Geometry check sheet. Reference: the model listing, model coordinates, mm. A direction names the side the tool comes from. Coordinates: 2 decimals unless noted, no trailing zeros. Order: outer loops, then holes, each group sorted by start corner. A loop starts at its lowest first (then second) coordinate and runs counter-clockwise, first axis right, second up. Notation, with made-up numbers: M 59.25,-28 L 86.25,-28 A19 cw 86.25,-1 Z; hole C 42.5,60 d1. An arc over 180 degrees is marked long. One line per item, written item: value. Start each with the question number.
1) Sectioned sample at B-B, the plane y = 107. Enter the section's corners in (x, z), then the cut area to 3 significant figures.
2) Go/stop test with flat-tipped pins: P1, Ø8.5, axis at x = 22.37, y = 47.5, coming from the +Z side; P2, Ø4, axis at x = 21.5, y = 47, coming from the +Z side; P3, Ø3, axis at y = 26, z = -41.5, coming from the -X side; P4, Ø2, axis at x = -45.13, z = -49.4, coming from the +Y side. Record where each tip stops, or that it passes through.
3) Thickness scan on L1, parallel to X at y = 6.5, z = -19.5; L2, parallel to X at y = 23, z = -22; L3, parallel to X at y = 47, z = -58. Record the ranges inside material, lowest first. Write a range as from..to.
4) Sectioned sample at A-A, the plane z = -35. State how many separate pieces and enclosed holes the cut face has, then the cut area to 3 significant figures.
5) Access from +Z, -Z, +X, -X, +Y, -Y to the whole of each face (thin tool, end or side, straight path). Record for faces 5 (the flat face through (-58.627, 44, -44)), 6 (the flat face through (21, 124, -55.901)), 7 (the flat face through (-66.627, 46, -43)), 8 (the flat face through (-63, 97, -49.401)).
6) Sectioned sample at D-D, the plane y = 18.5. Enter the section's corners in (x, z), then the cut area to 3 significant figures.
7) Draft check along Y on faces 1 (the flat face through (-16.7, -1.5, 7.1)), 2 (the flat face through (-64, 124, -55.901)), 3 (the flat face through (22, 97, -49.401)), 4 (the flat face through (-43, -10, -40)). Enter one of: pulls with the +Y half, pulls with the -Y half, needs draft (parallel to the pull), parting line crosses it, or undercut.
8) Sectioned sample at C-C, the plane x = -9. Enter the section's corners in (y, z), then the cut area to 3 significant figures.
```python
from build123d import *

# Parameters (mm, degrees)
SKETCH1_W           = 100
SKETCH1_H           = 70
SKETCH1_R           = 1.375
SKETCH1_R_2         = 27.5
BOSS_EXTRUDE1_DEPTH = 10
SKETCH3_W           = 8
SKETCH3_H           = 70
BOSS_EXTRUDE2_DEPTH = 55
CHAMFER1_SIZE       = 60
CHAMFER2_SIZE       = 3.5
SKETCH5_W           = 8
SKETCH5_H           = 10
BOSS_EXTRUDE3_DEPTH = 85
CUT_EXTRUDE1_START  = -3.5
SKETCH4_R           = 2.6
CUT_EXTRUDE1_DEPTH  = 169.016070813
SKETCH4_3_R         = 1.375
CUT_EXTRUDE2_DEPTH  = 172.516070813
CHAMFER3_SIZE       = 1


with BuildPart() as part:
    # Sketch1 → Boss-Extrude1 (new body)
    with BuildSketch(Plane(origin=(0, 0, 0), x_dir=(1, 0, 0), z_dir=(0, 1, 0))):
        with Locations((-20.126760563, 24.401408451)):
            Rectangle(SKETCH1_W, SKETCH1_H)
        with Locations(Location((-45.126760563, 49.401408451, 0), (0, 0, 270))):
            Circle(SKETCH1_R, mode=Mode.SUBTRACT)
        with Locations(Location((4.873239437, 49.401408451, 0), (0, 0, 270))):
            Circle(SKETCH1_R, mode=Mode.SUBTRACT)
        with Locations(Location((4.873239437, -0.598591549, 0), (0, 0, 270))):
            Circle(SKETCH1_R, mode=Mode.SUBTRACT)
        with Locations(Location((-45.126760563, -0.598591549, 0), (0, 0, 270))):
            Circle(SKETCH1_R, mode=Mode.SUBTRACT)
        with Locations(Location((-20.126760563, 24.401408451, 0), (0, 0, 270))):
            Circle(SKETCH1_R_2, mode=Mode.SUBTRACT)
    extrude(amount=-BOSS_EXTRUDE1_DEPTH)

    # Sketch3 → Boss-Extrude2 (add)
    with BuildSketch(Plane(origin=(0, 0, 0), x_dir=(1, 0, 0), z_dir=(0, 1, 0))):
        with Locations((-62.626760563, 24.401408451)):
            Rectangle(SKETCH3_W, SKETCH3_H)
        with Locations((22.373239437, 24.401408451)):
            Rectangle(SKETCH3_W, SKETCH3_H)
    extrude(amount=BOSS_EXTRUDE2_DEPTH)

    # Chamfer1
    chamfer1_edges = [part.edges().sort_by_distance(p)[0] for p in [
        (-62.626760563, 55, 10.598591549),
    ]]
    chamfer(chamfer1_edges, length=CHAMFER1_SIZE)

    # Chamfer2
    chamfer2_edges = [part.edges().sort_by_distance(p)[0] for p in [
        (26.373239437, 0, -26.901408451),
        (-66.626760563, 0, -26.901408451),
    ]]
    chamfer(chamfer2_edges, length=CHAMFER2_SIZE - 0.0001)  # a hair under: the kernel refuses the full size

    # Sketch5 → Boss-Extrude3 (add)
    with BuildSketch(Plane(origin=(0, 55, 0), x_dir=(1, 0, 0), z_dir=(0, 1, 0))):
        with Locations((-62.626760563, 54.401408451)):
            Rectangle(SKETCH5_W, SKETCH5_H)
        with Locations((22.373239437, 54.401408451)):
            Rectangle(SKETCH5_W, SKETCH5_H)
    extrude(amount=BOSS_EXTRUDE3_DEPTH)

    # Sketch4 → Cut-Extrude1 (cut, through all)
    with BuildSketch(Plane(origin=(0, 0, -59.401408451), x_dir=(-1, 0, 0), z_dir=(0, 0, -1)).offset(CUT_EXTRUDE1_START)):
        with Locations((-22.373239437, 47.5)):
            Circle(SKETCH4_R)
        with Locations((62.626760563, 47.5)):
            Circle(SKETCH4_R)
        with Locations((62.626760563, 7.5)):
            Circle(SKETCH4_R)
        with Locations((-22.373239437, 7.5)):
            Circle(SKETCH4_R)
        with Locations((-22.373239437, 125)):
            Circle(SKETCH4_R)
        with Locations((62.626760563, 125)):
            Circle(SKETCH4_R)
    extrude(amount=-CUT_EXTRUDE1_DEPTH, mode=Mode.SUBTRACT)

    # Sketch4<3> → Cut-Extrude2 (cut, through all)
    with BuildSketch(Plane(origin=(0, 0, -59.401408451), x_dir=(-1, 0, 0), z_dir=(0, 0, -1))):
        with Locations((-22.373239437, 47.5)):
            Circle(SKETCH4_3_R)
        with Locations((-22.373239437, 7.5)):
            Circle(SKETCH4_3_R)
        with Locations((62.626760563, 47.5)):
            Circle(SKETCH4_3_R)
        with Locations((62.626760563, 7.5)):
            Circle(SKETCH4_3_R)
        with Locations((-22.373239437, 125)):
            Circle(SKETCH4_3_R)
        with Locations((62.626760563, 125)):
            Circle(SKETCH4_3_R)
    extrude(amount=-CUT_EXTRUDE2_DEPTH, mode=Mode.SUBTRACT)

    # Chamfer3
    chamfer3_edges = [part.edges().sort_by_distance(p)[0] for p in [
        (-66.626760563, 29.24995, -23.651358451),
        (-66.626760563, 97.5, -49.401408451),
        (-58.626760563, 97.5, -49.401408451),
        (26.373239437, 97.5, -49.401408451),
        (18.373239437, 97.5, -49.401408451),
        (26.373239437, 29.24995, -23.651358451),
        (18.373239437, 27.5, -21.901408451),
        (-58.626760563, 27.5, -21.901408451),
    ]]
    chamfer(chamfer3_edges, length=CHAMFER3_SIZE)


solid = part.part
```
Final values:
1. outline: M -66.63,-59.4 L -58.63,-59.4 L -58.63,-50.4 L -59.63,-49.4 L -65.63,-49.4 L -66.63,-50.4 Z; M 18.37,-59.4 L 26.37,-59.4 L 26.37,-50.4 L 25.37,-49.4 L 19.37,-49.4 L 18.37,-50.4 Z
1. area: 158 mm^2
2. P1: stops at z = -37.65
2. P2: stops at z = -39.4
2. P3: stops at x = -66.63
2. P4: passes through
3. L1: x = -66.63..-65.03, -60.23..-58.63, 18.37..19.97, 24.77..26.37
3. L2: x = -66.63..-58.63, 18.37..26.37
3. L3: x = -66.63..-63.91, -61.35..-58.63, 18.37..21.09, 23.65..26.37
4. separate pieces: 2
4. enclosed holes: 2
4. area: 1,110 mm^2
5. face 5: +Z, -Z, +Y
5. face 6: +Z
5. face 7: +Z, -Z, -X, +Y
5. face 8: +Z, +X, -X, +Y
6. outline: M -66.63,-59.4 L -58.63,-59.4 L -58.63,-14.32 L -59.63,-12.9 L -65.63,-12.9 L -66.63,-14.32 Z; M 18.37,-59.4 L 26.37,-59.4 L 26.37,-14.32 L 25.37,-12.9 L 19.37,-12.9 L 18.37,-14.32 Z
6. area: 741 mm^2
7. face 1: pulls with the +Y half
7. face 2: undercut
7. face 3: needs draft
7. face 4: pulls with the -Y half
8. outline: M -10,-59.4 L 0,-59.4 L 0,-49.55 L -10,-49.55 Z; M -10,0.75 L 0,0.75 L 0,5.6 L -5,10.6 L -10,10.6 Z
8. area: 185 mm^2
